Here's how the part is built. I have some questions about the finished solid (model axes, mm). Face numbers are marked on the shaded views. A direction names the side the tool comes from. Give positions to 0.01 mm unless a question says otherwise; leave off trailing zeros. Return JSON: item names as keys, results as strings.
from build123d import *


with BuildPart() as part:
    # Sketch2 → Revolve1 (revolve)
    with BuildSketch(Plane.XY):
        Polygon((-35, 20), (35, 20), (35, 54), (26.5, 54), (26.5, 120.622540289), (80, 145.57), (80, 185), (69.641016151, 185), (60.980762114, 200), (50.980762114, 200), (42.320508076, 185), (32.320508076, 185), (23.660254038, 200), (13.660254038, 200), (5, 185), (-5, 185), (-13.660254038, 200), (-23.660254038, 200), (-32.320508076, 185), (-42.320508076, 185), (-50.980762114, 200), (-60.980762114, 200), (-69.641016151, 185), (-80, 185), (-80, 145.57), (-26.5, 120.622540289), (-26.5, 54), (-35, 54), align=None)
    revolve(axis=Axis((-192.57069662, 0, 0), (1, 0, 0)))


solid = part.part
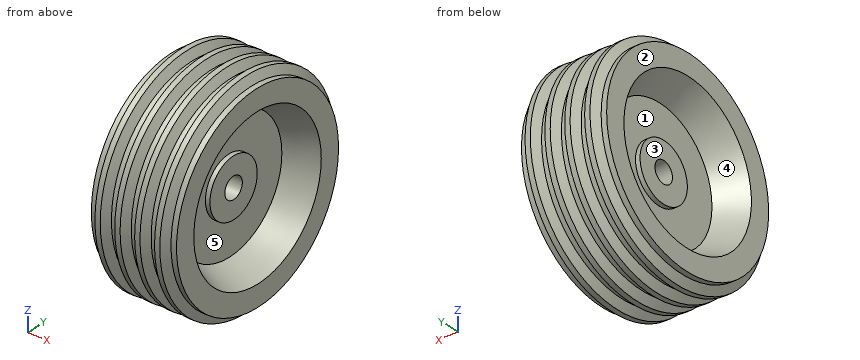
1. Which directions (+Z, -Z, +X, -X, +Y, -Y) give clear straight access to the entire face, cutting with the end or side of a thin tool? Please do the marked faces 4 and 5.
Taken from the geometry:
{"face 4": "-X", "face 5": "+X"}
2. If I drill on line 1 (Z direction, x = -15, y = 0); line 2 (Z direction, x = -66.5, y = 12); line 3 (Y direction, x = -73, z = -8.5), over which ranges is the centre line in solid material (lowest first)? Write a range as [from, to].
Taken from the geometry:
{"line 1": "z = [-200, -20], [20, 200]", "line 2": "z = [-190.06, -138.76], [138.76, 190.06]", "line 3": "y = [-184.8, -142.05], [142.05, 184.8]"}
3. For pin 1 Ø12 at (x, y) = (37, 94) entering from +Z; pin 2 Ø10 at (x, z) = (57, 152) entering from -Y; pin 3 Ø10 at (x, z) = (-10, 80) entering from +Y, each with a flat end and sliding along its axis, tell me the tip position at first contact or that it passes through.
Taken from the geometry:
{"pin 1": "stops at z = 162.73", "pin 2": "stops at y = -135.61", "pin 3": "stops at y = 184.75"}
4. If we mould it in two halves opening along Y, with no side actions, what happens to the marked faces 1, 2 and 3? For each: released by +Y, released by -Y, zero draft, split by the parting line, or undercut.
Taken from the geometry:
{"face 1": "undercut", "face 2": "zero draft", "face 3": "undercut"}
